```python
from build123d import *

# Parameters (mm, degrees)
F2_R    = 2
F3_SIZE = 2


with BuildPart() as f1:
    # F0 (on Front) → F1 (revolve)
    with BuildSketch(Plane.XZ):
        Polygon((0, 26.836595), (0, 0), (86.229056, 0), (86.229056, 43.847769), (47.220673, 43.847769), (47.220673, 10.998603), (19.944135, 10.998603), (19.944135, 26.836595), align=None)
    revolve(axis=Axis((43.114528, 0, 0), (1, 0, 0)))

    # F2
    f2_edges = [f1.edges().sort_by_distance(p)[0] for p in [
        (0, 0, -26.836595),
    ]]
    fillet(f2_edges, radius=F2_R)

    # F3
    f3_edges = [f1.edges().sort_by_distance(p)[0] for p in [
        (47.220673, 0, -43.847769),
    ]]
    chamfer(f3_edges, length=F3_SIZE)


solid = f1.part
```
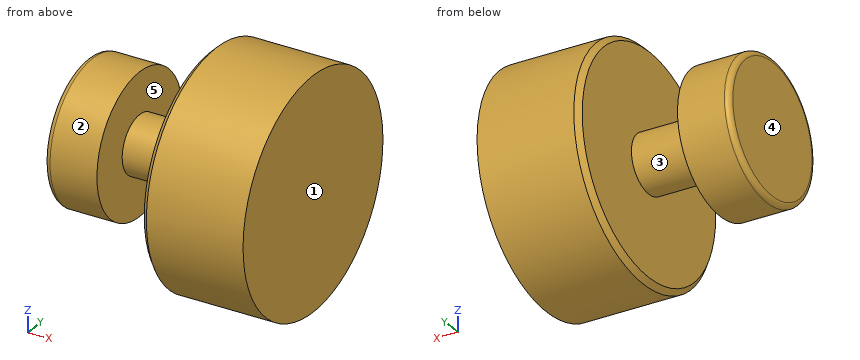
CAD build for the part. Positions are in the model's coordinates, mm. Face numbers are marked on the shaded views. A direction names the side the tool comes from. Round coordinates to 2 decimals unless told otherwise and drop trailing zeros. Write each loop counter-clockwise with the first axis right and the second up, starting at its lowest first coordinate (ties: lowest second). Pieces come first, ordered by that corner, then holes.
Item 1: Drop flat-ended pins along their axis: pin 1 Ø1.5 at (x, y) = (65, -22.5) entering from -Z; pin 2 Ø1.5 at (x, z) = (61, 17.5) entering from -Y; pin 3 Ø3 at (y, z) = (28.5, -15.5) entering from -X. Give the stop position or say it passes through.
Filled in:
pin 1: stops at z = -38.07
pin 2: stops at y = -40.52
pin 3: stops at x = 47.22
Item 2: Band-saw the part on A-A on y = 0. Write the cut outline in (x, z).
Filled in:
outline: (0, -24.84) arc R2 ccw to (2, -26.84) - (19.94, -26.84) - (19.94, -11) - (47.22, -11) - (47.22, -41.85) - (49.22, -43.85) - (86.23, -43.85) - (86.23, 43.85) - (49.22, 43.85) - (47.22, 41.85) - (47.22, 11) - (19.94, 11) - (19.94, 26.84) - (2, 26.84) arc R2 ccw to (0, 24.84) - close
Item 3: Mould opens along X. For the marked faces 1, 2 and 3 say: released by +X, released by -X, zero draft, split by the parting line, or undercut.
Filled in:
face 1: released by +X
face 2: zero draft
face 3: undercut
Item 4: Band-saw the part on C-C on x = 9. Write the cut outline in (y, z), then the cut area to 3 significant figures.
Filled in:
outline: circle Ø53.67 at (0, 0)
area: 2,260 mm2
Item 5: Band-saw the part on D-D on x = 51.5. Write the cut outline in (y, z).
Filled in:
outline: circle Ø87.7 at (0, 0)
Item 6: Drill centre lines: L1, parallel to X at y = 13, z = -4; L2, parallel to X at y = 15, z = -30.5; L3, parallel to Z at x = 37.5, y = -8. Where is each one in solid material? Low to high.
Filled in:
L1: x = 0 to 19.94, 47.22 to 86.23
L2: x = 47.22 to 86.23
L3: z = -7.55 to 7.55
Item 7: Tool access for the marked faces 4 and 5: list every direction of +Z, -Z, +X, -X, +Y, -Y with a clear straight run to the whole face (end or side of a thin tool).
Filled in:
face 4: +Z, -Z, -X, +Y, -Y
face 5: none
